```python
from build123d import *

# Parameters (mm, degrees)
F0_W          = 11.43
F0_H          = 11.43
F1_DEPTH      = 30.48
F3_DEPTH      = 12.7
F3_DEPTH_BACK = 25.4


with BuildPart() as f1:
    # F0 (on Front) → F1 (new body)
    with BuildSketch(Plane.XZ):
        with BuildLine():
            Line((12.7, 38.1), (1.27, 38.1))
            ThreePointArc((1.27, 38.1), (0, 36.83), (-1.27, 38.1))
            Line((-1.27, 38.1), (-12.7, 38.1))
            Line((-12.7, 38.1), (-12.7, -26.67))
            Line((-12.7, -26.67), (-1.27, -26.67))
            Line((-1.27, -26.67), (-1.27, 25.4))
            Line((-1.27, 25.4), (1.27, 25.4))
            Line((1.27, 25.4), (1.27, -26.67))
            Line((1.27, -26.67), (12.7, -26.67))
            Line((12.7, -26.67), (12.7, 38.1))
        make_face()
        with BuildLine():
            ThreePointArc((-1.27, 38.1), (0, 36.83), (1.27, 38.1))
            Line((1.27, 38.1), (0.909717055, 38.1))
            Line((0.909717055, 38.1), (0.909717055, 37.846))
            Line((0.909717055, 37.846), (0.5819871133, 37.846))
            ThreePointArc((0.5819871133, 37.846), (0.4490128061, 37.6509871939), (0.254, 37.5180128867))
            Line((0.254, 37.5180128867), (0.254, 37.3829295754))
            Line((0.254, 37.3829295754), (-0.254, 37.3829295754))
            Line((-0.254, 37.3829295754), (-0.254, 37.5180128867))
            ThreePointArc((-0.254, 37.5180128867), (-0.4490128061, 37.6509871939), (-0.5819871133, 37.846))
            Line((-0.5819871133, 37.846), (-0.909717055, 37.846))
            Line((-0.909717055, 37.846), (-0.909717055, 38.1))
            Line((-0.909717055, 38.1), (-1.27, 38.1))
        make_face()
        with Locations((-6.985, -32.385)):
            Rectangle(F0_W, F0_H)
        with Locations((-18.415, -32.385)):
            Rectangle(F0_W, F0_H)
        with Locations((6.985, -32.385)):
            Rectangle(F0_W, F0_H)
        with Locations((18.415, -32.385)):
            Rectangle(F0_W, F0_H)
        with BuildLine():
            Line((0.909717055, 38.1), (1.27, 38.1))
            ThreePointArc((1.27, 38.1), (0, 39.37), (-1.27, 38.1))
            Line((-1.27, 38.1), (-0.909717055, 38.1))
            Line((-0.909717055, 38.1), (-0.909717055, 38.354))
            Line((-0.909717055, 38.354), (-0.5819871133, 38.354))
            ThreePointArc((-0.5819871133, 38.354), (-0.4490128061, 38.5490128061), (-0.254, 38.6819871133))
            Line((-0.254, 38.6819871133), (-0.254, 38.8170704246))
            Line((-0.254, 38.8170704246), (0.254, 38.8170704246))
            Line((0.254, 38.8170704246), (0.254, 38.6819871133))
            ThreePointArc((0.254, 38.6819871133), (0.4490128061, 38.5490128061), (0.5819871133, 38.354))
            Line((0.5819871133, 38.354), (0.909717055, 38.354))
            Line((0.909717055, 38.354), (0.909717055, 38.1))
        make_face()
        with BuildLine():
            Line((-0.635, 38.1), (-0.909717055, 38.1))
            Line((-0.909717055, 38.1), (-0.909717055, 37.846))
            Line((-0.909717055, 37.846), (-0.5819871133, 37.846))
            ThreePointArc((-0.5819871133, 37.846), (-0.6216055087, 37.9702633763), (-0.635, 38.1))
        make_face()
        with BuildLine():
            Line((-0.909717055, 38.354), (-0.909717055, 38.1))
            Line((-0.909717055, 38.1), (-0.635, 38.1))
            ThreePointArc((-0.635, 38.1), (-0.6216055087, 38.2297366237), (-0.5819871133, 38.354))
            Line((-0.5819871133, 38.354), (-0.909717055, 38.354))
        make_face()
        with BuildLine():
            ThreePointArc((-0.254, 38.6819871133), (-0.4490128061, 38.5490128061), (-0.5819871133, 38.354))
            Line((-0.5819871133, 38.354), (-0.254, 38.354))
            Line((-0.254, 38.354), (-0.254, 38.6819871133))
        make_face()
        with BuildLine():
            Line((0.254, 38.354), (0.5819871133, 38.354))
            ThreePointArc((0.5819871133, 38.354), (0.4490128061, 38.5490128061), (0.254, 38.6819871133))
            Line((0.254, 38.6819871133), (0.254, 38.354))
        make_face()
        with BuildLine():
            Line((0.635, 38.1), (0.909717055, 38.1))
            Line((0.909717055, 38.1), (0.909717055, 38.354))
            Line((0.909717055, 38.354), (0.5819871133, 38.354))
            ThreePointArc((0.5819871133, 38.354), (0.6216055087, 38.2297366237), (0.635, 38.1))
        make_face()
        with BuildLine():
            Line((0.909717055, 37.846), (0.909717055, 38.1))
            Line((0.909717055, 38.1), (0.635, 38.1))
            ThreePointArc((0.635, 38.1), (0.6216055087, 37.9702633763), (0.5819871133, 37.846))
            Line((0.5819871133, 37.846), (0.909717055, 37.846))
        make_face()
        with BuildLine():
            ThreePointArc((0.254, 37.5180128867), (0.4490128061, 37.6509871939), (0.5819871133, 37.846))
            Line((0.5819871133, 37.846), (0.254, 37.846))
            Line((0.254, 37.846), (0.254, 37.5180128867))
        make_face()
        with BuildLine():
            Line((0.254, 37.3829295754), (0.254, 37.5180128867))
            ThreePointArc((0.254, 37.5180128867), (0, 37.465), (-0.254, 37.5180128867))
            Line((-0.254, 37.5180128867), (-0.254, 37.3829295754))
            Line((-0.254, 37.3829295754), (0.254, 37.3829295754))
        make_face()
        with BuildLine():
            ThreePointArc((-0.254, 38.6819871133), (0, 38.735), (0.254, 38.6819871133))
            Line((0.254, 38.6819871133), (0.254, 38.8170704246))
            Line((0.254, 38.8170704246), (-0.254, 38.8170704246))
            Line((-0.254, 38.8170704246), (-0.254, 38.6819871133))
        make_face()
        with BuildLine():
            Line((-0.254, 37.846), (-0.5819871133, 37.846))
            ThreePointArc((-0.5819871133, 37.846), (-0.4490128061, 37.6509871939), (-0.254, 37.5180128867))
            Line((-0.254, 37.5180128867), (-0.254, 37.846))
        make_face()
    extrude(amount=F1_DEPTH)

    # F2 (on face) → F3 (cut, two sides)
    with BuildSketch(Plane.XY.offset(38.1)) as f3_sk:
        Polygon((12.7, -27.94), (12.7, -2.54), (-6.985, -2.54), (-26.67, -2.54), (-26.67, -27.94), align=None)
    extrude(amount=-F3_DEPTH, mode=Mode.SUBTRACT)
    extrude(f3_sk.sketch, amount=F3_DEPTH_BACK, mode=Mode.SUBTRACT)


solid = f1.part
```
Check sheet for the modelled part. Datum: model origin and axes. Units: mm. A direction names the side the tool comes from. Round coordinates to 2 decimals unless told otherwise and drop trailing zeros. Order: outer loops, then holes, each group sorted by start corner. A loop starts at its lowest first (then second) coordinate and runs counter-clockwise, first axis right, second up. Notation, with made-up numbers: (43, 45) -> (55, 45) arc R35 cw to (55, 84) -> close; hole circle Ø11 at (75.5, -4). An arc over 180 degrees is marked (long way). One line per item, written item: value. Start each with the question number.
Q1. Cross-section at D-D (z = 22). Record the boundary of the cut face in (x, y).
Q2. Cross-section at A-A (z = -32.5). Record the boundary of the cut face in (x, y).
Q3. Set-up check for faces 4 (the face through (7, -15, 25.4)), 5 (the face through (0, -29, 25.4)), 6 (the face through (18, -15, -26.67)), 7 (the face through (-12.7, -15, -1)): record each of +Z, -Z, +X, -X, +Y, -Y from which the full face is reachable in a straight line by a thin tool's end or side.
Q4. Mould release check, pull along X, two halves, no side actions. Record for faces 1 (the face through (-7, -15, 25.4)), 2 (the face through (-1.27, -15, -7)), 3 (the face through (-24.13, -15, -32)): pulls with the +X half, pulls with the -X half, needs draft (parallel to the pull), parting line crosses it, or undercut.
Q5. Thickness scan on line 1 (X direction, y = -8, z = 11.5); line 2 (X direction, y = -28, z = -30); line 3 (Z direction, x = 10, y = -11). Record the ranges inside material, lowest first.
Q6. Cross-section at C-C (x = 8). Record the boundary of the cut face in (y, z).
Q7. Cross-section at B-B (y = -13.5). Record the boundary of the cut face in (x, z).
Q8. Gauge pin test, flat ends, axial feed: pin 1 Ø9 at (y, z) = (-18.5, 4) entering from -X; pin 2 Ø0.8 at (x, y) = (-6.5, -29.5) entering from +Z; pin 3 Ø3 at (x, y) = (-10, -13) entering from +Z. Record the tip position at first contact, or that the pin passes through.
Completed:
1. outline: (-12.7, -30.48) -> (-1.27, -30.48) -> (-1.27, 0) -> (-12.7, 0) -> close; (1.27, -30.48) -> (12.7, -30.48) -> (12.7, 0) -> (1.27, 0) -> close
2. outline: (-24.13, -30.48) -> (-1.27, -30.48) -> (-1.27, 0) -> (-24.13, 0) -> close; (1.27, -30.48) -> (24.13, -30.48) -> (24.13, 0) -> (1.27, 0) -> close
3. face 4: +Z, +X, -X
3. face 5: -Z, +Y, -Y
3. face 6: +Z, +X, +Y, -Y
3. face 7: +Z, -X, +Y, -Y
4. face 1: needs draft
4. face 2: undercut
4. face 3: pulls with the -X half
5. line 1: x = -12.7 to -1.27, 1.27 to 12.7
5. line 2: x = -24.13 to -1.27, 1.27 to 24.13
5. line 3: z = -38.1 to 25.4
6. outline: (-30.48, -38.1) -> (0, -38.1) -> (0, 38.1) -> (-2.54, 38.1) -> (-2.54, 25.4) -> (-27.94, 25.4) -> (-27.94, 38.1) -> (-30.48, 38.1) -> close
7. outline: (-24.13, -38.1) -> (-1.27, -38.1) -> (-1.27, 25.4) -> (-12.7, 25.4) -> (-12.7, -26.67) -> (-24.13, -26.67) -> close; (1.27, -38.1) -> (24.13, -38.1) -> (24.13, -26.67) -> (12.7, -26.67) -> (12.7, 25.4) -> (1.27, 25.4) -> close
8. pin 1: stops at x = -12.7
8. pin 2: stops at z = 38.1
8. pin 3: stops at z = 25.4
